Source: CAD feature listing. Evaluate the final solid. Frame: model axes, mm. A direction names the side the tool comes from. Give positions to 0.01 mm unless a question says otherwise; leave off trailing zeros. Loops run counter-clockwise (first coordinate to the right, second up) from the corner with the lowest first, then second, coordinate; pieces in that order, holes last. Notation, with made-up numbers: M 30.5,61 L 71.5,61 A9 cw 71.5,70 Z; hole C 10,32 d3. An arc over 180 degrees is marked long. Answer in a Markdown table with one row per item.
```python
from build123d import *

# Parameters (mm, degrees)
SKETCH1_R           = 1.1
BOSS_EXTRUDE1_DEPTH = 1.5
BOSS_EXTRUDE2_DEPTH = 25.5
BOSS_EXTRUDE4_DEPTH = 2


with BuildPart() as part:
    # Sketch1 → Boss-Extrude1 (new body)
    with BuildSketch(Plane.XY):
        with BuildLine():
            Line((65, 15), (65, 5))
            Line((65, 5), (47.403, 5.0215))
            ThreePointArc((47.403, 5.0215), (45.32489976, 5.287606245), (43.379, 6.064))
            Line((43.379, 6.064), (9.7, 27.063))
            ThreePointArc((9.7, 27.063), (6.483564725, 30.296790106), (5.042, 34.624))
            Line((5.042, 34.624), (5, 50))
            Line((5, 50), (5.042, 65.376))
            ThreePointArc((5.042, 65.376), (6.483564725, 69.703209894), (9.7, 72.937))
            Line((9.7, 72.937), (43.379, 93.936))
            ThreePointArc((43.379, 93.936), (45.32489976, 94.712393755), (47.403, 94.9785))
            Line((47.403, 94.9785), (65, 95))
            Line((65, 95), (65, 85))
            Line((65, 85), (65, 82))
            Line((65, 82), (40.367460006, 82))
            Line((40.367460006, 82), (40.367460006, 77.700799702))
            Line((40.367460006, 77.700799702), (37.816539887, 76.993905452))
            Line((37.816539887, 76.993905452), (37.261948992, 78.995219046))
            Line((37.261948992, 78.995219046), (26.063497318, 75.891977576))
            Line((26.063497318, 75.891977576), (26.618088213, 73.890663982))
            Line((26.618088213, 73.890663982), (13.092809655, 70.14262751))
            Line((13.092809655, 70.14262751), (10.021, 65.77301003))
            Line((10.021, 65.77301003), (10.021, 34.22698997))
            Line((10.021, 34.22698997), (13.092809655, 29.85737249))
            Line((13.092809655, 29.85737249), (26.618088213, 26.109336018))
            Line((26.618088213, 26.109336018), (26.063497318, 24.108022424))
            Line((26.063497318, 24.108022424), (37.261948992, 21.004780954))
            Line((37.261948992, 21.004780954), (37.816539887, 23.006094548))
            Line((37.816539887, 23.006094548), (40.367460006, 22.299200298))
            Line((40.367460006, 22.299200298), (40.367460006, 18))
            Line((40.367460006, 18), (65, 18))
            Line((65, 18), (65, 15))
        make_face()
        with Locations((32.343, 84.089)):
            Circle(SKETCH1_R, mode=Mode.SUBTRACT)
        with Locations((14.76, 72.68)):
            Circle(SKETCH1_R, mode=Mode.SUBTRACT)
        with Locations((14.76, 27.32)):
            Circle(SKETCH1_R, mode=Mode.SUBTRACT)
        with Locations((32.343, 15.911)):
            Circle(SKETCH1_R, mode=Mode.SUBTRACT)
        Polygon((47.33363322, 83.065556795), (55.303190804, 82.368310853), (56.261903975, 93.326452532), (48.29234639, 94.023698474), align=None, mode=Mode.SUBTRACT)
        Polygon((58.032899046, 86.65175686), (61.864724228, 86.65175686), (61.864724228, 88.544627634), (64.004574654, 88.544627634), (64.004574654, 91.546423221), (61.864868117, 91.546423221), (61.864868117, 93.072013731), (58.032899046, 93.072013731), align=None, mode=Mode.SUBTRACT)
        Polygon((56.261903975, 6.673547468), (48.29234639, 5.976301526), (47.33363322, 16.934443205), (55.303190804, 17.631689147), align=None, mode=Mode.SUBTRACT)
        Polygon((58.032899046, 13.34824314), (61.864724228, 13.34824314), (61.864724228, 11.455372366), (64.004574654, 11.455372366), (64.004574654, 8.453576779), (61.864868117, 8.453576779), (61.864868117, 6.927986269), (58.032899046, 6.927986269), align=None, mode=Mode.SUBTRACT)
    extrude(amount=BOSS_EXTRUDE1_DEPTH)

    # Sketch2 → Boss-Extrude2 (add)
    with BuildSketch(Plane.XY.offset(1.5)):
        Polygon((26.618088213, 26.109336018), (26.063497318, 24.108022424), (24.063497318, 24.662249304), (24.618088213, 26.663562898), align=None)
        Polygon((37.261948992, 21.004780954), (37.816539887, 23.006094548), (39.816539887, 22.451867667), (39.261948992, 20.450554074), align=None)
        Polygon((39.816539887, 77.548132333), (39.261948992, 79.549445926), (37.261948992, 78.995219046), (37.816539887, 76.993905452), align=None)
        Polygon((26.063497318, 75.891977576), (24.063497318, 75.337750696), (24.618088213, 73.336437102), (26.618088213, 73.890663982), align=None)
        Polygon((47.340340229, 18), (51.96241715, 18), (51.96241715, 17.488205474), (47.340340229, 17.083826141), align=None)
        Polygon((48.330167759, 5.770045696), (51.96241715, 6.087826341), (51.96241715, 5.015929308), (48.330167759, 5.020367187), (48.330167759, 5.551877825), align=None)
        Polygon((48.330167759, 94.979632813), (48.330167759, 94.448122175), (48.330167759, 94.229954304), (51.96241715, 93.912173659), (51.96241715, 94.984070692), align=None)
        Polygon((47.340340229, 82.916173859), (51.96241715, 82.511794526), (51.96241715, 82), (47.340340229, 82), align=None)
    extrude(amount=BOSS_EXTRUDE2_DEPTH)

    # Sketch4 → Boss-Extrude4 (add)
    with BuildSketch(Plane.XY.offset(27)):
        Polygon((48.330167759, 5.020367187), (48.330167759, 5.770045696), (47.340340229, 17.083826141), (47.340340229, 18), (51.96241715, 18), (51.96241715, 17.488205474), (51.96241715, 5.015929308), align=None)
        Polygon((24.618088213, 26.663562898), (39.816539887, 22.451867667), (39.261948992, 20.450554074), (24.063497318, 24.662249304), align=None)
        Polygon((51.96241715, 82.511794526), (51.96241715, 94.984070692), (48.330167759, 94.979632813), (48.330167759, 94.229954304), (47.340340229, 82.916173859), (47.340340229, 82), (51.96241715, 82), align=None)
        Polygon((39.261948992, 79.549445926), (24.063497318, 75.337750696), (24.618088213, 73.336437102), (39.816539887, 77.548132333), align=None)
    extrude(amount=BOSS_EXTRUDE4_DEPTH)


solid = part.part
```
Q1. Ray query, probe 1 along Z at (x, y) = (34, 85.5); probe 2 along Y at (x, z) = (14.76, 0.3); probe 3 along X at (y, z) = (22, 21.5). Return the intervals inside material, ascending. Write a range as from..to.
Values follow:
| item | result |
|---|---|
| probe 1 | 0..1.5 |
| probe 2 | 23.91..26.22, 28.42..29.4, 70.6..71.58, 73.78..76.09 |
| probe 3 | 37.54..39.69 |
Q2. Mould query, pull axis X, two halves, no side actions, for faces 1 (the cylindrical face through (31.47, 83.42, 0.74)), 2 (the flat face through (32, 23, 29)), 3 (the flat face through (26.337, 74.905, 13.311)). Classes: +X half, -X half, draft (parallel to the pull), parting line (faces both ways), or undercut.
Values follow:
| item | result |
|---|---|
| face 1 | undercut |
| face 2 | draft |
| face 3 | +X half |
Q3. Contact query for flat-ended pins moving along their axis: pin 1 Ø3.5 at (x, y) = (50, 12.5) entering from -Z; pin 2 Ø8 at (y, z) = (28.5, 7) entering from -X; pin 3 Ø0.8 at (y, z) = (80.5, 1) entering from +X. Output: stop coordinate, or through.
Values follow:
| item | result |
|---|---|
| pin 1 | z = 27 |
| pin 2 | x = 24.06 |
| pin 3 | x = 40.37 |
Q4. Section query A-A (z = 5.5). Give the number of separate pieces and of enclosed holes in the cut face, plus the area to 3 significant figures.
Values follow:
| item | result |
|---|---|
| separate pieces | 8 |
| enclosed holes | 0 |
| area | 30.5 mm^2 |
Q5. Reachability of faces 4 (the flat face through (49.619, 82.717, 14.072)), 5 (the flat face through (31.741, 77.465, 0.74)), 6 (the flat face through (24.337, 74.351, 15.058)), 7 (the flat face through (51.962, 94.3, 20.3)) from +Z, -Z, +X, -X, +Y, -Y: full face, straight path, thin tool, end or side. Return the list, or none.
Values follow:
| item | result |
|---|---|
| face 4 | +X |
| face 5 | -Z |
| face 6 | +Z, -X |
| face 7 | +Z, +X, +Y, -Y |
Q6. Section query C-C (x = 14.76). Output: boundary loops of the cut face in (y, z).
Values follow:
| item | result |
|---|---|
| outline | M 23.91,0 L 26.22,0 L 26.22,1.5 L 23.91,1.5 Z; M 28.42,0 L 29.4,0 L 29.4,1.5 L 28.42,1.5 Z; M 70.6,0 L 71.58,0 L 71.58,1.5 L 70.6,1.5 Z; M 73.78,0 L 76.09,0 L 76.09,1.5 L 73.78,1.5 Z |
Q7. Section query B-B (x = 22). Output: boundary loops of the cut face in (y, z).
Values follow:
| item | result |
|---|---|
| outline | M 19.39,0 L 27.39,0 L 27.39,1.5 L 19.39,1.5 Z; M 72.61,0 L 80.61,0 L 80.61,1.5 L 72.61,1.5 Z |
